For this review, take the finished solid that the model builds, in its own axes (mm). A direction names the side the tool comes from. Round coordinates to 2 decimals unless told otherwise and drop trailing zeros. Write each loop counter-clockwise with the first axis right and the second up, starting at its lowest first coordinate (ties: lowest second). Pieces come first, ordered by that corner, then holes. Notation, with made-up numbers: (75, 69.25) - (109, 69.25) arc R17 ccw to (109, 83.25) - close; hole circle Ø7 at (56, 29.5). An arc over 180 degrees is marked (long way). One line per item, written item: value. Start each with the question number.
Q1. Add section A-A on y = 15. Write out the cut boundary in (x, z), and give its area (3 significant figures).
Q2. For probe 1 along Y at (x, z) = (9.75, 6.75); probe 2 along X at (y, z) = (14, 10.5); probe 3 along Z at (x, y) = (4.25, 19.5), list the stretches that pass through material, from the lowest coordinate up.
Q3. Add section C-C on z = 11. Write out the cut boundary in (x, y), and give its area (3 significant figures).
Q4. Tool access review of faces 1 (the face through (4, 19, 19.05)), 2 (the face through (18.288, 19, 9)), 3 (the face through (0, 23, 10)): name each direction out of +Z, -Z, +X, -X, +Y, -Y from which nothing blocks a thin tool from reaching the whole face with its end or side.
Q5. Add section D-D on x = 5.75. Write out the cut boundary in (y, z), and give its area (3 significant figures).
Q6. Clearance check with flat-ended pins moving along their axes: pin 1 Ø1.6 at (x, z) = (20.5, 9) entering from -Y; pin 2 Ø14 at (x, z) = (7.5, 14) entering from -Y; pin 3 Ø2.5 at (x, y) = (2.5, 18) entering from +Z. State where each tip first meets the part, or that it passes through.
Q7. Add section B-B on x = 19. Write out the cut boundary in (y, z).
```python
from build123d import *

# Parameters (mm, degrees)
F0_W     = 25.4
F0_H     = 6.35
F1_DEPTH = 38.1
F4_DEPTH = 25.4
F6_DEPTH = 12.7


with BuildPart() as f1:
    # F0 (on Front) → F1 (new body)
    with BuildSketch(Plane.XZ):
        with Locations((12.7, 3.175)):
            Rectangle(F0_W, F0_H)
    extrude(amount=-F1_DEPTH)

    # F3 (on offset) → F4 (join)
    with BuildSketch(Plane.XZ.offset(-12.7)):
        Polygon((0, 25.4), (0, 6.35), (25.4, 6.35), align=None)
    extrude(amount=-F4_DEPTH)

    # F5 (on face) → F6 (cut)
    with BuildSketch(Plane.XZ.offset(-12.7)):
        Polygon((8.4666666667, 19.05), (0, 25.4), (0, 19.05), align=None)
        Polygon((18.288, 6.35), (25.4, 6.35), (18.288, 11.684), align=None)
    extrude(amount=-F6_DEPTH, mode=Mode.SUBTRACT)


solid = f1.part
```
Result set:
1. outline: (0, 0) - (25.4, 0) - (25.4, 6.35) - (18.29, 6.35) - (18.29, 11.68) - (8.47, 19.05) - (0, 19.05) - close
1. area: 357 mm^2
2. probe 1: y = 12.7 to 38.1
2. probe 2: x = 0 to 18.29
2. probe 3: z = 0 to 19.05
3. outline: (0, 12.7) - (18.29, 12.7) - (18.29, 25.4) - (19.2, 25.4) - (19.2, 38.1) - (0, 38.1) - close
3. area: 476 mm^2
4. face 1: +Z, +X, -X, -Y
4. face 2: +Z, +X, -Y
4. face 3: +Z, -Z, -X, +Y, -Y
5. outline: (0, 0) - (38.1, 0) - (38.1, 21.09) - (25.4, 21.09) - (25.4, 19.05) - (12.7, 19.05) - (12.7, 6.35) - (0, 6.35) - close
5. area: 590 mm^2
6. pin 1: stops at y = 25.4
6. pin 2: stops at y = 12.7
6. pin 3: stops at z = 19.05
7. outline: (0, 0) - (38.1, 0) - (38.1, 11.15) - (25.4, 11.15) - (25.4, 6.35) - (0, 6.35) - close
